Could you check a few things on this model? Use its own coordinates, in mm. A direction names the side the tool comes from. Coordinates: 2 decimals unless noted, no trailing zeros. Loops run counter-clockwise (first coordinate to the right, second up) from the corner with the lowest first, then second, coordinate; pieces in that order, holes last.
1) If I drill on line 1 along Y through (x, z) = (-23, 3.65); line 2 along X through (y, z) = (-32, 6.5); line 3 along X through (y, z) = (-28, 5.25), over which ranges is the centre line in solid material (lowest first)?
2) Thinking about a two-plate mould opening in X: for faces 1 (the face through (-36.6, 26.07, 0.99)), 2 (the face through (-49.089, 38.196, 1.014)), 3 (the face through (48.772, -28.377, 7.071)), which applies, released by +X, released by -X, zero draft, split by the parting line, or undercut?
3) Imagine slicing it at D-D on x = -36. Please give me the cut outline in (y, z), plus the area to 3 significant figures.
4) Imagine slicing it at C-C on x = -23. Please give me the cut outline in (y, z), plus the area to 3 significant figures.
5) For faces 4 (the face through (48.828, 27.112, 9.827)), 5 (the face through (-23, -33, 2)), 6 (the face through (-46.8, -29, 5)), 7 (the face through (0, -27.5, 1)), which set-ups out of +Z, -Z, +X, -X, +Y, -Y let a thin tool reach every point of the face, with its end or its side?
6) Will these pins go through, and if not, where does the flat tip stop? P1, Ø1.6, axis at x = -23.5, y = -33.5, coming from the +Z side; P2, Ø7, axis at x = -23.5, y = -33, coming from the +Z side; P3, Ø1.2, axis at x = 49.5, z = 3.5, coming from the +Y side; P4, Ø8, axis at x = 28.5, y = -23, coming from the -Z side.
7) Imagine slicing it at B-B on z = 3.25. Give the number of separate pieces and of enclosed holes in the cut face, plus the area to 3 significant figures.
8) Imagine slicing it at A-A on y = -13. Please give me the cut outline in (x, z), plus the area to 3 significant figures.
```python
from build123d import *

# Parameters (mm, degrees)
SKETCH_W        = 101.6
SKETCH_H        = 80
PAD_DEPTH       = 2
SKETCH001_W     = 4
SKETCH001_H     = 8
PAD001_DEPTH    = 9
SKETCH002_R     = 1.625
POCKET_DEPTH    = 101.6
SKETCH003_R     = 1.625
POCKET001_DEPTH = 101.6
SKETCH004_R     = 3.2
SKETCH004_R_2   = 1.6
PAD002_DEPTH    = 6
SKETCH005_W     = 76.2
SKETCH005_H     = 55
POCKET002_DEPTH = 4
FILLET_R        = 3.9
FILLET001_R     = 6
FILLET002_R     = 5


with BuildPart() as part:
    # Sketch → Pad (new body)
    with BuildSketch(Plane.XY):
        Rectangle(SKETCH_W, SKETCH_H)
    extrude(amount=PAD_DEPTH)

    # Sketch001 (on Face6 of Pad) → Pad001 (join)
    with BuildSketch(Plane.XY.offset(2)):
        with Locations((-48.8, 30)):
            Rectangle(SKETCH001_W, SKETCH001_H)
        with Locations((48.8, 30)):
            Rectangle(SKETCH001_W, SKETCH001_H)
        with Locations((48.8, -30)):
            Rectangle(SKETCH001_W, SKETCH001_H)
        with Locations((-48.8, -30)):
            Rectangle(SKETCH001_W, SKETCH001_H)
    extrude(amount=PAD001_DEPTH)

    # Sketch002 (on Face8 of Pad001) → Pocket (cut)
    with BuildSketch(Plane(origin=(-50.8, 0, 0), x_dir=(0, -1, 0), z_dir=(-1, 0, 0))):
        with Locations((-30, 7)):
            Circle(SKETCH002_R)
    extrude(amount=-POCKET_DEPTH, mode=Mode.SUBTRACT)

    # Sketch003 (on Face7 of Pocket) → Pocket001 (cut)
    with BuildSketch(Plane(origin=(-50.8, 0, 0), x_dir=(0, -1, 0), z_dir=(-1, 0, 0))):
        with Locations((30, 7)):
            Circle(SKETCH003_R)
    extrude(amount=-POCKET001_DEPTH, mode=Mode.SUBTRACT)

    # Sketch004 (on Face5 of Pocket001) → Pad002 (join)
    with BuildSketch(Plane.XY.offset(2)):
        with Locations((-23, 33)):
            Circle(SKETCH004_R)
        with Locations((-23, 33)):
            Circle(SKETCH004_R_2, mode=Mode.SUBTRACT)
        with Locations((23, 33)):
            Circle(SKETCH004_R)
        with Locations((23, 33)):
            Circle(SKETCH004_R_2, mode=Mode.SUBTRACT)
        with Locations((23, -33)):
            Circle(SKETCH004_R)
        with Locations((23, -33)):
            Circle(SKETCH004_R_2, mode=Mode.SUBTRACT)
        with Locations((-23, -33)):
            Circle(SKETCH004_R)
        with Locations((-23, -33)):
            Circle(SKETCH004_R_2, mode=Mode.SUBTRACT)
    extrude(amount=PAD002_DEPTH)

    # Sketch005 (on Face5 of Pad002) → Pocket002 (cut)
    with BuildSketch(Plane.XY.offset(2)):
        Rectangle(SKETCH005_W, SKETCH005_H)
    extrude(amount=-POCKET002_DEPTH, mode=Mode.SUBTRACT)

    # Fillet
    fillet_edges = [part.edges().sort_by_distance(p)[0] for p in [
        (48.8, -34, 11),
        (48.8, -26, 11),
        (48.8, 26, 11),
        (48.8, 34, 11),
        (-48.8, 34, 11),
        (-48.8, 26, 11),
        (-48.8, -26, 11),
        (-48.8, -34, 11),
    ]]
    fillet(fillet_edges, radius=FILLET_R)

    # Fillet001
    fillet001_edges = [part.edges().sort_by_distance(p)[0] for p in [
        (-50.8, -40, 1),
        (50.8, -40, 1),
        (-50.8, 40, 1),
        (50.8, 40, 1),
    ]]
    fillet(fillet001_edges, radius=FILLET001_R)

    # Fillet002
    fillet002_edges = [part.edges().sort_by_distance(p)[0] for p in [
        (38.1, 27.5, 1),
        (38.1, -27.5, 1),
        (-38.1, 27.5, 1),
        (-38.1, -27.5, 1),
    ]]
    fillet(fillet002_edges, radius=FILLET002_R)


solid = part.part
```
Filled in:
1. line 1: y = -36.2 to -34.6, -31.4 to -29.8, 29.8 to 31.4, 34.6 to 36.2
1. line 2: x = -50.8 to -46.8, -26.04 to -24.25, -21.75 to -19.96, 19.96 to 21.75, 24.25 to 26.04, 46.8 to 50.8
1. line 3: x = -50.8 to -46.8, 46.8 to 50.8
2. face 1: undercut
2. face 2: released by -X
2. face 3: zero draft
3. outline: (-40, 0) - (-26.57, 0) - (-26.57, 2) - (-40, 2) - close; (26.57, 0) - (40, 0) - (40, 2) - (26.57, 2) - close
3. area: 53.7 mm2
4. outline: (-40, 0) - (-27.5, 0) - (-27.5, 2) - (-29.8, 2) - (-29.8, 8) - (-31.4, 8) - (-31.4, 2) - (-34.6, 2) - (-34.6, 8) - (-36.2, 8) - (-36.2, 2) - (-40, 2) - close; (27.5, 0) - (40, 0) - (40, 2) - (36.2, 2) - (36.2, 8) - (34.6, 8) - (34.6, 2) - (31.4, 2) - (31.4, 8) - (29.8, 8) - (29.8, 2) - (27.5, 2) - close
4. area: 88.4 mm2
5. face 4: +Z, +X, -X
5. face 5: +Z
5. face 6: +Z, +Y, -Y
5. face 7: +Z, -Z
6. P1: stops at z = 2
6. P2: stops at z = 8
6. P3: stops at y = 34
6. P4: passes through
7. separate pieces: 8
7. enclosed holes: 4
7. area: 225 mm2
8. outline: (-50.8, 0) - (-38.1, 0) - (-38.1, 2) - (-50.8, 2) - close; (38.1, 0) - (50.8, 0) - (50.8, 2) - (38.1, 2) - close
8. area: 50.8 mm2
